from build123d import *

# Parameters (mm, degrees)
F0_W     = 76.2
F0_H     = 31.75
F1_DEPTH = 698.5
F2_W     = 508
F2_H     = 19.05
F3_DEPTH = 12.7
F4_W     = 76.2
F4_H     = 31.75
F5_DEPTH = 12.7


with BuildPart() as f1:
    # F0 (on Front) → F1 (new body)
    with BuildSketch(Plane.XZ):
        with Locations((38.066154, 16.090209)):
            Rectangle(F0_W, F0_H)
    extrude(amount=F1_DEPTH)

    # F2 (on face) → F3 (cut)
    with BuildSketch(Plane(origin=(-0.033846, 0, 0), x_dir=(0, -1, 0), z_dir=(-1, 0, 0))):
        with Locations((342.9, 9.740209)):
            Rectangle(F2_W, F2_H)
    extrude(amount=-F3_DEPTH, mode=Mode.SUBTRACT)

    # F4 (on face) → F5 (cut)
    with BuildSketch(Plane.XY.offset(31.965209)):
        with Locations((38.066154, -574.675)):
            Rectangle(F4_W, F4_H)
        with Locations((38.066154, -111.125)):
            Rectangle(F4_W, F4_H)
    extrude(amount=-F5_DEPTH, mode=Mode.SUBTRACT)


solid = f1.part
Work out the finished part from the listing and answer in its coordinate system (mm). A direction names the side the tool comes from. Give positions to 0.01 mm unless a question says otherwise; leave off trailing zeros. Loops run counter-clockwise (first coordinate to the right, second up) from the corner with the lowest first, then second, coordinate; pieces in that order, holes last. Notation, with made-up numbers: (88, 43) -> (128, 43) arc R11 cw to (128, 51) -> close; hole circle Ø5 at (-2.75, 19.5). An arc over 180 degrees is marked (long way). Use a Markdown table: item, result. Add a question column.
1) The part is cut by section A-A, the plane z = 26. Determine the outline of the cut face in (x, y), plus the area to 3 significant figures.
2) The part is cut by section B-B, the plane y = -428.5. Determine the outline of the cut face in (x, z).
3) Which of the six approach directions +Z, -Z, +X, -X, +Y, -Y give full straight-line access (tool end or side, diameter ignored) to faces 1 (the flat face through (38, -644, 31.965)), 2 (the flat face through (44, -574, 19.265)), 3 (the flat face through (6, -88.9, 10))?
4) Each of these flat-tipped pins is pushed along its axis until it touches: P1, Ø4, axis at x = 3.5, y = -342, coming from the -Z side; P2, Ø9.5, axis at x = 33, y = -114.5, coming from the +Z side; P3, Ø8, axis at y = -416, z = 14.5, coming from the -X side. Where does it stop, or does it pass through?
5) For a pull along Y with two mould halves and no side action, classify faces 4 (the flat face through (38, -590.55, 26)), 5 (the flat face through (6, -340, 19.265)), 6 (the flat face through (38, -698.5, 16)), 7 (the flat face through (38, -340, 31.965)) as +Y half, -Y half, draft (parallel to the pull), parting line (faces both ways), or undercut.
6) The part is cut by section C-C, the plane x = 37. Determine the outline of the cut face in (y, z).
7) Consider line 1 along Y through (x, z) = (29.5, 28.5); line 2 along X through (y, z) = (-243.5, 13); line 3 along Y through (x, z) = (11, 13). Determine where each line is inside the solid, lowest interval first.
Reported:
| question | item | result |
|---|---|---|
| 1 | outline | (-0.03, -698.5) -> (76.17, -698.5) -> (76.17, -590.55) -> (-0.03, -590.55) -> close; (-0.03, -558.8) -> (76.17, -558.8) -> (76.17, -127) -> (-0.03, -127) -> close; (-0.03, -95.25) -> (76.17, -95.25) -> (76.17, 0) -> (-0.03, 0) -> close |
| 1 | area | 48,400 mm^2 |
| 2 | outline | (-0.03, 19.27) -> (12.67, 19.27) -> (12.67, 0.22) -> (76.17, 0.22) -> (76.17, 31.97) -> (-0.03, 31.97) -> close |
| 3 | face 1 | +Z, +X, -X, +Y, -Y |
| 3 | face 2 | +Z, +X, -X |
| 3 | face 3 | -Z, -X |
| 4 | P1 | stops at z = 19.27 |
| 4 | P2 | stops at z = 19.27 |
| 4 | P3 | stops at x = 12.67 |
| 5 | face 4 | undercut |
| 5 | face 5 | undercut |
| 5 | face 6 | -Y half |
| 5 | face 7 | draft |
| 6 | outline | (-698.5, 0.22) -> (0, 0.22) -> (0, 31.97) -> (-95.25, 31.97) -> (-95.25, 19.27) -> (-127, 19.27) -> (-127, 31.97) -> (-558.8, 31.97) -> (-558.8, 19.27) -> (-590.55, 19.27) -> (-590.55, 31.97) -> (-698.5, 31.97) -> close |
| 7 | line 1 | y = -698.5 to -590.55, -558.8 to -127, -95.25 to 0 |
| 7 | line 2 | x = 12.67 to 76.17 |
| 7 | line 3 | y = -698.5 to -596.9, -88.9 to 0 |
